For this review, take the finished solid that the model builds, in its own axes (mm). A direction names the side the tool comes from. Round coordinates to 2 decimals unless told otherwise and drop trailing zeros. Write each loop counter-clockwise with the first axis right and the second up, starting at its lowest first coordinate (ties: lowest second). Pieces come first, ordered by that corner, then holes. Notation, with made-up numbers: (-21.75, 36.25) - (17.25, 36.25) arc R9 cw to (17.25, 48.25) - close; hole circle Ø2 at (-14, 57). An arc over 180 degrees is marked (long way). One line per item, written item: value. Start each with the question number.
Q1. For probe 1 along X at (y, z) = (0.5, 52); probe 2 along X at (y, z) = (2.5, 39); probe 3 along X at (y, z) = (3.45, 77.61), list the stretches that pass through material, from the lowest coordinate up.
Q2. Add section C-C on x = 99.5. Write out the cut boundary in (y, z), and give its area (3 significant figures).
Q3. Clearance check with flat-ended pins moving along their axes: pin 1 Ø11 at (x, z) = (51, 67.5) entering from +Y; pin 2 Ø1.8 at (x, z) = (104, 0) entering from -Y; pin 3 Ø1.5 at (y, z) = (1.5, 98.5) entering from -X; pin 4 Ø2.5 at (y, z) = (2.5, 106) entering from +X. State where each tip first meets the part, or that it passes through.
Q4. Mouldability with a two-part tool opening along Z and no side actions: class faces 1 (the face through (127, 2, 39)), 2 (the face through (90, 3, 45)), 3 (the face through (52, 2, 115.002)) as +Z half, -Z half, draft (parallel to the pull), parting line (faces both ways), or undercut.
Q5. Add section D-D on z = 106. Write out the cut boundary in (x, y).
Q6. Add section B-B on y = 3.85. Write out the cut boundary in (x, z).
Q7. Add section A-A on z = 30. Write out the cut boundary in (x, y), and give its area (3 significant figures).
Q8. Tool access review of faces 4 (the face through (14, 3, 45)), 5 (the face through (36, 1, 103)), 6 (the face through (34, 3, 68)): name each direction out of +Z, -Z, +X, -X, +Y, -Y from which nothing blocks a thin tool from reaching the whole face with its end or side.
```python
from build123d import *

# Parameters (mm, degrees)
BOSS_EXTRUDE1_DEPTH          = 5
F_3_0_3_DIAMETER_HOLE1_D     = 3
F_3_0_3_DIAMETER_HOLE1_DEPTH = 6
F_3_0_3_DIAMETER_HOLE1_TIP   = 0.901290929
SKETCH6_W                    = 36
SKETCH6_H                    = 120
CUT_EXTRUDE1_DEPTH           = 3
SKETCH9_W                    = 20
SKETCH9_H                    = 45
CUT_EXTRUDE3_DEPTH           = 172.404214254
SKETCH10_W                   = 2
SKETCH10_H                   = 25
CUT_EXTRUDE4_DEPTH           = 172.404214254
FILLET3_R                    = 2


with BuildPart() as part:
    # Sketch3 → Boss-Extrude1 (new body)
    with BuildSketch(Plane(origin=(0, 0, 0), x_dir=(1, 0, 0), z_dir=(0, 1, 0))):
        Polygon((32.540994622, -115.001759396), (71.460246245, -115.001759396), (127, -59.462005641), (127, -18.529510204), (109.123269601, 8.998240604), (-5.122028734, 8.998240604), (-23, -18.531420972), (-23, -59.460764774), align=None)
    extrude(amount=BOSS_EXTRUDE1_DEPTH)

    # Ø3.0 (3) Diameter Hole1
    with Locations(Plane(origin=(0, 5, 0), x_dir=(1, 0, 0), z_dir=(0, 1, 0))):
        with Locations((95.841240867, -77.61), (8.16, -77.61), (103.998195646, -0.001759396), (0.003045221, -0.001759396)):
            Hole(F_3_0_3_DIAMETER_HOLE1_D / 2, depth=F_3_0_3_DIAMETER_HOLE1_DEPTH)
            with Locations((0, 0, -(F_3_0_3_DIAMETER_HOLE1_DEPTH + F_3_0_3_DIAMETER_HOLE1_TIP / 2))):  # 118° drill point
                Cone(0, F_3_0_3_DIAMETER_HOLE1_D / 2, F_3_0_3_DIAMETER_HOLE1_TIP, mode=Mode.SUBTRACT)

    # Sketch6 → Cut-Extrude1 (cut)
    with BuildSketch(Plane(origin=(0, 5, 0), x_dir=(1, 0, 0), z_dir=(0, 1, 0))):
        with Locations((52, -53.001759396)):
            Rectangle(SKETCH6_W, SKETCH6_H)
    extrude(amount=-CUT_EXTRUDE1_DEPTH, mode=Mode.SUBTRACT)

    # Sketch9 → Cut-Extrude3 (cut, through all)
    with BuildSketch(Plane(origin=(0, 5, 0), x_dir=(1, 0, 0), z_dir=(0, 1, 0))):
        with Locations((4, -45.11)):
            Rectangle(SKETCH9_W, SKETCH9_H)
    cut_extrude3 = extrude(amount=-CUT_EXTRUDE3_DEPTH, mode=Mode.SUBTRACT)

    # Mirror1: Cut-Extrude3 across plane
    add(cut_extrude3.mirror(Plane(origin=(52, 0, 0), x_dir=(0, 0, 1), z_dir=(1, 0, 0))), mode=Mode.SUBTRACT)

    # Sketch10 → Cut-Extrude4 (cut, through all)
    with BuildSketch(Plane(origin=(0, 5, 0), x_dir=(1, 0, 0), z_dir=(0, 1, 0))):
        with Locations((35, -102.501759396)):
            Rectangle(SKETCH10_W, SKETCH10_H)
        with Locations((69, -102.501759396)):
            Rectangle(SKETCH10_W, SKETCH10_H)
    extrude(amount=-CUT_EXTRUDE4_DEPTH, mode=Mode.SUBTRACT)

    # Fillet3
    fillet3_edges = [part.edges().sort_by_distance(p)[0] for p in [
        (52, 5, 113.001759396),
    ]]
    fillet(fillet3_edges, radius=FILLET3_R - 0.0001)  # a hair under: the kernel refuses the full size


solid = part.part
```
Result set:
1. probe 1: x = -23 to -6, 14 to 90, 110 to 127
1. probe 2: x = -23 to -6, 14 to 34, 70 to 90, 110 to 127
1. probe 3: x = -4.85 to 6.66, 9.66 to 34, 70 to 94.34, 97.34 to 108.85
2. outline: (0, -9) - (5, -9) - (5, 22.61) - (0, 22.61) - close; (0, 67.61) - (5, 67.61) - (5, 86.96) - (0, 86.96) - close
2. area: 255 mm^2
3. pin 1: stops at y = 2
3. pin 2: passes through
3. pin 3: stops at x = 15.29
3. pin 4: stops at x = 81.71
4. face 1: draft
4. face 2: undercut
4. face 3: +Z half
5. outline: (23.54, 0) - (34, 0) - (34, 5) - (23.54, 5) - close; (36, 0) - (68, 0) - (68, 2) - (36, 2) - close; (70, 0) - (80.46, 0) - (80.46, 5) - (70, 5) - close
6. outline: (-23, 18.53) - (-5.12, -9) - (109.12, -9) - (127, 18.53) - (127, 59.46) - (71.46, 115) - (70, 115) - (70, -7) - (34, -7) - (34, 115) - (32.54, 115) - (-23, 59.46) - close; (36, 113.19) - (68, 113.19) - (68, 115) - (36, 115) - close; hole (-6, 22.61) - (14, 22.61) - (14, 67.61) - (-6, 67.61) - close; hole circle Ø3 at (0, 0); hole circle Ø3 at (8.16, 77.61); hole (90, 22.61) - (110, 22.61) - (110, 67.61) - (90, 67.61) - close; hole circle Ø3 at (95.84, 77.61); hole circle Ø3 at (104, 0)
7. outline: (-23, 0) - (-6, 0) - (-6, 5) - (-23, 5) - close; (14, 0) - (90, 0) - (90, 5) - (70, 5) - (70, 2) - (34, 2) - (34, 5) - (14, 5) - close; (110, 0) - (127, 0) - (127, 5) - (110, 5) - close
7. area: 442 mm^2
8. face 4: +Y, -Y
8. face 5: +Z, +Y, -Y
8. face 6: +Z, +Y
